Can you work these out from the model? Positions are in its coordinate system, mm. Coordinates: 2 decimals unless noted, no trailing zeros. Order: outer loops, then holes, each group sorted by start corner. A loop starts at its lowest first (then second) coordinate and runs counter-clockwise, first axis right, second up. Notation, with made-up numbers: (-8.75, 71) -> (4.25, 71) arc R22 cw to (4.25, 82) -> close; hole circle Ø4 at (86, 36.5). An arc over 180 degrees is marked (long way). Use a Markdown table: item, result. Add a question column.
1. Suppose I cut it at C-C, the plane z = 22.5. List the corners of the cut face in (x, y) for me.
2. If I drill on line 1 along Z through (x, y) = (-95, 4.5); line 2 along X through (y, z) = (5.25, 31); line 3 along Z through (x, y) = (-144.5, 4), over which ranges is the centre line in solid material (lowest first)? Write a range as from..to.
3. For pin 1 Ø3 at (y, z) = (2, -28) entering from +X; pin 2 Ø0.6 at (y, z) = (2, -19.5) entering from -X; pin 3 Ø2 at (x, y) = (-103.5, 2.5) entering from +Z; pin 4 Ø3 at (x, z) = (-109.5, -7) entering from -Y, each with a flat end and sliding along its axis, tell me the tip position at first contact or that it passes through.
4. Suppose I cut it at A-A, the plane z = -21. List the corners of the cut face in (x, y) for me.
5. Suppose I cut it at B-B, the plane x = -108. List the corners of the cut face in (y, z) for me, then the cut area to 3 significant figures.
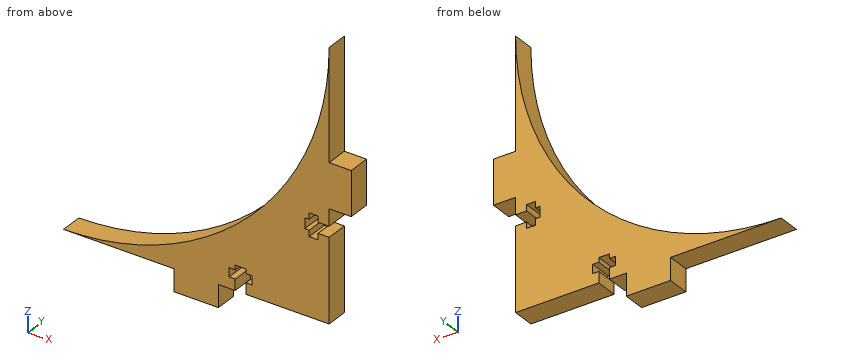
```python
from build123d import *

# Parameters (mm, degrees)
BOSS_EXTRUDE1_DEPTH = 6.35


with BuildPart() as part:
    # Sketch1 → Boss-Extrude1 (new body)
    with BuildSketch(Plane(origin=(0, 0, 0), x_dir=(1, 0, 0), z_dir=(0, 1, 0))):
        with BuildLine():
            Line((-172.086243064, 25.662027693), (-140.336243064, 25.662027693))
            Line((-140.336243064, 25.662027693), (-140.336243064, 32.012027693))
            Line((-140.336243064, 32.012027693), (-127.636243064, 32.012027693))
            Line((-127.636243064, 32.012027693), (-127.636243064, 25.662027693))
            Line((-127.636243064, 25.662027693), (-122.810172742, 25.662027693))
            Line((-122.810172742, 25.662027693), (-122.810172742, 22.487027693))
            Line((-122.810172742, 22.487027693), (-124.562772742, 22.487027693))
            Line((-124.562772742, 22.487027693), (-124.562772742, 19.947027693))
            Line((-124.562772742, 19.947027693), (-122.810172742, 19.947027693))
            Line((-122.810172742, 19.947027693), (-122.810172742, 18.677027693))
            Line((-122.810172742, 18.677027693), (-119.762313386, 18.677027693))
            Line((-119.762313386, 18.677027693), (-119.762313386, 19.947027693))
            Line((-119.762313386, 19.947027693), (-118.009713386, 19.947027693))
            Line((-118.009713386, 19.947027693), (-118.009713386, 22.487027693))
            Line((-118.009713386, 22.487027693), (-119.762313386, 22.487027693))
            Line((-119.762313386, 22.487027693), (-119.762313386, 25.662027693))
            Line((-119.762313386, 25.662027693), (-95.886243064, 25.662027693))
            Line((-95.886243064, 25.662027693), (-95.886243064, 1.785957371))
            Line((-95.886243064, 1.785957371), (-99.061243064, 1.785957371))
            Line((-99.061243064, 1.785957371), (-99.061243064, 3.538557371))
            Line((-99.061243064, 3.538557371), (-101.601243064, 3.538557371))
            Line((-101.601243064, 3.538557371), (-101.601243064, 1.785957371))
            Line((-101.601243064, 1.785957371), (-102.871243064, 1.785957371))
            Line((-102.871243064, 1.785957371), (-102.871243064, -1.261901985))
            Line((-102.871243064, -1.261901985), (-101.601243064, -1.261901985))
            Line((-101.601243064, -1.261901985), (-101.601243064, -3.014501985))
            Line((-101.601243064, -3.014501985), (-99.061243064, -3.014501985))
            Line((-99.061243064, -3.014501985), (-99.061243064, -1.261901985))
            Line((-99.061243064, -1.261901985), (-95.886243064, -1.261901985))
            Line((-95.886243064, -1.261901985), (-95.886243064, -6.087972307))
            Line((-95.886243064, -6.087972307), (-89.536243064, -6.087972307))
            Line((-89.536243064, -6.087972307), (-89.536243064, -18.787972307))
            Line((-89.536243064, -18.787972307), (-95.886243064, -18.787972307))
            Line((-95.886243064, -18.787972307), (-95.886243064, -50.537972307))
            ThreePointArc((-95.886243064, -50.537972307), (-118.204706338, 3.34356442), (-172.086243064, 25.662027693))
        make_face()
    extrude(amount=BOSS_EXTRUDE1_DEPTH)


solid = part.part
```
Worked out:
| question | item | result |
|---|---|---|
| 1 | outline | (-101.23, 0) -> (-95.89, 0) -> (-95.89, 6.35) -> (-101.23, 6.35) -> close |
| 2 | line 1 | z = 6.09..18.79 |
| 2 | line 2 | x = -98.43..-95.89 |
| 2 | line 3 | z = -25.66..-20.49 |
| 3 | pin 1 | stops at x = -127.64 |
| 3 | pin 2 | stops at x = -142.78 |
| 3 | pin 3 | stops at z = 19.49 |
| 3 | pin 4 | stops at y = 0 |
| 4 | outline | (-145.84, 0) -> (-124.56, 0) -> (-124.56, 6.35) -> (-145.84, 6.35) -> close; (-118.01, 0) -> (-95.89, 0) -> (-95.89, 6.35) -> (-118.01, 6.35) -> close |
| 5 | outline | (0, -25.66) -> (6.35, -25.66) -> (6.35, 9.31) -> (0, 9.31) -> close |
| 5 | area | 222 mm² |
